Design review of the part built by this model. Coordinates are the model's own, in mm. A direction names the side the tool comes from. Coordinates: 2 decimals unless noted, no trailing zeros. Answer as a JSON object with one key per item and string values. Group by question number.
1. Machinability: for faces 3 (the cylindrical face through (-55.105, 17.226, -2.059)), 4 (the flat face through (48.514, 34.3, -0.7)), 5 (the cylindrical face through (0.679, 19.064, -0.976)), which of the approach directions +Z, -Z, +X, -X, +Y, -Y give a long, thin tool a straight path to every point of the face, cutting with its end or side? Answer none if there is none.
2. Draft analysis for pull direction Z (two halves, no side actions). For faces 1 (the cylindrical face through (55.105, 17.226, 2.059)), 2 (the flat face through (-61.514, 18, -5)), state which applies: +Z half, -Z half, draft (parallel to the pull), parting line (faces both ways), or undercut.
3. To check wall thickness, follow probe 1 along Y at (x, z) = (-0.5, 0); probe 2 along Y at (x, z) = (-58, 0); probe 3 along X at (y, z) = (25, -8.5). State the ranges of each line that lie inside material, in increasing order.
4. Insertion check: pin 1 (8 mm diameter, centred on x = -29.5, z = 10, fed in from -Y); pin 2 (8 mm diameter, centred on x = -17, y = 41, fed in from -Z); pin 3 (6 mm diameter, centred on y = 20.5, z = 13, fed in from +X); pin 4 (11.5 mm diameter, centred on y = 26.5, z = 0, fed in from +X). Each pin has a flat end and moves straight along its axis. Give the tip position at first contact, or say it passes through.
Autodesk Inventor part; units mm, degrees
ref_plane "Work Plane1" through (0, 0, 0) normal (0, -0.8660254, 0.5) x (1, 0, 0)
ref_plane "YZ Plane" through (0, 0, 0) normal (1, 0, 0) x (0, 1, 0)
ref_plane "XZ Plane" through (0, 0, 0) normal (0, 1, 0) x (-1, 0, 0)
ref_plane "Work Plane1" through (0, 0, 0) normal (0, -0.8660254, 0.5) x (1, 0, 0)
sketch "Sketch1" plane through (0, 0, 0) normal (0, -0.8660254, 0.5) x (1, 0, 0)
  circle A0 centre (0, 0) radius 97 construction
  dimension "d1" = 194
sketch "Sketch2" plane through (0, 0, 0) normal (0, 0, 1) x (1, 0, 0)
  circle A0 centre (0, 26.5) radius 22 construction
  ellipse E0 centre (0, 0) end of major axis (97, 0) minor radius 48.5 construction
  line L0 (0, 26.5) -> (-61.5142, 26.5)
  line L1 (0, 37.5) -> (-61.5142, 37.5) construction
  line L2 (-61.5142, 37.5) -> (-61.5142, 26.5)
  line L3 (0, 0) -> (0, 48.5) construction
  line L4 (0, 26.5) -> (61.5142, 26.5)
  line L5 (61.5142, 37.5) -> (61.5142, 26.5)
  ellipse E1 centre (0, 0) end of major axis (97, 0) minor radius 48.5 (61.5142, 37.5) -> (-61.5142, 37.5) ccw
  dimension "d2" = 44
  dimension "d3" = 11
revolve "Revolution1" add sketch "Sketch2" angle 360 about axis through (0, 26.5, 0) along (1, 0, 0)
sketch "Sketch3" plane through (61.5142, 26.5, 0) normal (1, 0, 0) x (0, 0, -1)
  circle A0 centre (0, 0) radius 11
  circle A1 centre (0, 0) radius 9.5
  point P0 (0, -26.5)
  point P1 (0, 11)
  dimension "d5" = 19
extrude "Extrusion1" cut sketch "Sketch3" against normal blind 13 contours A1
sketch "Sketch4" plane through (-61.5142, 26.5, 0) normal (-1, 0, 0) x (0, 0, 1)
  circle A0 centre (0, 0) radius 9.5
  dimension "d8" = 19
extrude "Extrusion2" cut sketch "Sketch4" against normal blind 13
hole "Hole1" at (-48.5142, 26.5, 0) direction (1, 0, 0) diameter 15 end up to surface
properties part number "roller 8-19-6 bearing" material "Aluminum 6061"
Findings below:
{
 "1": {"face 3": "-X", "face 4": "+X", "face 5": "+X, -X"},
 "2": {"face 1": "undercut", "face 2": "draft"},
 "3": {"probe 1": "y = 4.5 to 19, 34 to 48.5", "probe 2": "y = 14.13 to 17, 36 to 38.87", "probe 3": "x = -48.51 to 48.51"},
 "4": {"pin 1": "stops at y = 7.58", "pin 2": "stops at z = -18.51", "pin 3": "stops at x = 60.73", "pin 4": "passes through"}
}
